CAD build for the part. Positions are in the model's coordinates, mm. Face numbers are marked on the shaded views. Give positions to 0.01 mm unless a question says otherwise; leave off trailing zeros. Use one line per item in the form item = value. Start each with the question number.
1) Drop flat-ended pins along their axis: P1, Ø6, axis at x = -9.5, z = 21, coming from the -Y side; P2, Ø12, axis at x = 11, y = 10, coming from the +Z side; P3, Ø12, axis at x = -7, z = 12.5, coming from the +Y side; P4, Ø2, axis at y = 12, z = 4, coming from the +X side. Give the stop position or say it passes through.
2) Probe line 1 (Y direction, x = 0, z = 23.25) (1 decimal); line 2 (X direction, y = 0, z = 7.25); line 3 (Y direction, x = 0, z = 4.75). List the from-to ranges inside material, lowest first.
3) Mould opens along Y. For the marked faces 1 and 2 say: pulls with the +Y half, pulls with the -Y half, needs draft (parallel to the pull), parting line crosses it, or undercut.
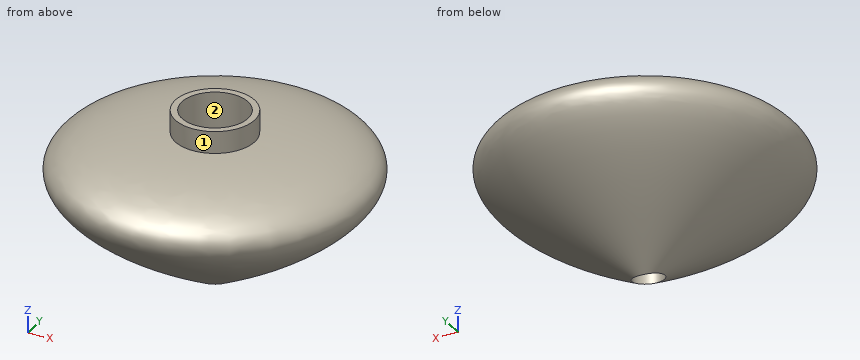
from build123d import *

# Parameters (mm, degrees)
F2_R     = 4.7625
F3_DEPTH = 9.525
F4_R     = 2.2225
F5_DEPTH = 14.605


# Not quite as in the source:
# - a feature names something its author has since deleted; it is built from what else it names


with BuildPart() as f1:
    # F0 (on Front) → F1 (revolve)
    with BuildSketch(Plane.XZ):
        with BuildLine():
            Line((0, 25.4), (0, 0))
            add(Edge.make_bspline(
                [(0, 0), (11.4623733169, 6.6295765693), (30.9367325307, 18.1147399727), (14.1349324056, 21.8956786186), (5.715, 22.225)],
                knots=[0, 0, 0, 0, 0.5612625766, 1, 1, 1, 1], degree=3))
            Line((5.715, 22.225), (5.715, 25.4))
            Line((5.715, 25.4), (0, 25.4))
        make_face()
    revolve(axis=Axis((0, 0, 12.7), (0, 0, -1)))

    # F2 (on face) → F3 (cut)
    with BuildSketch(Plane.XY.offset(25.4)):
        Circle(F2_R)
    extrude(amount=-F3_DEPTH, mode=Mode.SUBTRACT)

    # F4 (on Top) → F5 (cut)
    with BuildSketch(Plane.XY):
        with Locations((0, -0.9156785202)):
            Circle(F4_R)
    extrude(amount=F5_DEPTH, mode=Mode.SUBTRACT)


solid = f1.part
Result:
q1.P1 = -19.73
q1.P2 = 22.03
q1.P3 = 21.74
q1.P4 = through
q2.line_1 = -5.7 to -4.8, 4.8 to 5.7
q2.line_2 = -12.08 to -2.03, 2.03 to 12.08
q2.line_3 = -8.08 to -3.14, 1.31 to 8.08
q3.face_1 = parting line crosses it
q3.face_2 = undercut
